```python
from build123d import *

# Parameters (mm, degrees)
SKETCH1_R          = 9.525
BODY_DEPTH         = 6
SKETCH2_R          = 1.5
SKETCH2_R_2        = 5.5
SKETCH2_R_3        = 1.75
HOLES_DEPTH        = 6
FILLET1_R          = 10
FILLET2_R          = 40
SKETCH3_R          = 3.175
CUT_EXTRUDE2_DEPTH = 3


with BuildPart() as part:
    # Sketch1 → Body (new body)
    with BuildSketch(Plane(origin=(0, 0, 0), x_dir=(1, 0, 0), z_dir=(0, 1, 0))):
        with BuildLine():
            Line((45, -55), (15.965110713, -96.240145236))
            ThreePointArc((15.965110713, -96.240145236), (0, -104.525), (-15.965110713, -96.240145236))
            Line((-15.965110713, -96.240145236), (-45, -55))
            Line((-45, -55), (-45, 55))
            Line((-45, 55), (45, 55))
            Line((45, 55), (45, -55))
        make_face()
        with Locations(Location((0, -85, 0), (0, 0, 270))):
            Circle(SKETCH1_R, mode=Mode.SUBTRACT)
    extrude(amount=BODY_DEPTH)

    # Sketch2 → Holes (cut)
    with BuildSketch(Plane(origin=(0, 6, 0), x_dir=(1, 0, 0), z_dir=(0, 1, 0))):
        with Locations(Location((6.273420837, 45, 0), (0, 0, 270))):
            Circle(SKETCH2_R)
        with Locations(Location((-8.726579163, 45, 0), (0, 0, 270))):
            Circle(SKETCH2_R)
        with Locations(Location((-1.226579163, 45, 0), (0, 0, 270))):
            Circle(SKETCH2_R_2)
        with Locations(Location((37.5, -57.5, 0), (0, 0, 270))):
            Circle(SKETCH2_R_3)
        with Locations(Location((-37.5, -57.5, 0), (0, 0, 270))):
            Circle(SKETCH2_R_3)
        with Locations(Location((-37.5, -12.5, 0), (0, 0, 270))):
            Circle(SKETCH2_R_3)
        with Locations(Location((37.5, -12.5, 0), (0, 0, 270))):
            Circle(SKETCH2_R_3)
    extrude(amount=-HOLES_DEPTH, mode=Mode.SUBTRACT)

    # Fillet1
    fillet1_edges = [part.edges().sort_by_distance(p)[0] for p in [
        (45, 3, 55),
        (-45, 3, 55),
    ]]
    fillet(fillet1_edges, radius=FILLET1_R)

    # Fillet2
    fillet2_edges = [part.edges().sort_by_distance(p)[0] for p in [
        (-45, 3, -55),
        (45, 3, -55),
    ]]
    fillet(fillet2_edges, radius=FILLET2_R)

    # Sketch3 → Cut-Extrude2 (cut)
    with BuildSketch(Plane(origin=(0, 6, 0), x_dir=(1, 0, 0), z_dir=(0, 1, 0))):
        with Locations(Location((-37.5, -12.5, 0), (0, 0, 270))):
            Circle(SKETCH3_R)
        with Locations(Location((37.5, -12.5, 0), (0, 0, 270))):
            Circle(SKETCH3_R)
        with Locations(Location((37.5, -57.5, 0), (0, 0, 270))):
            Circle(SKETCH3_R)
        with Locations(Location((-37.5, -57.5, 0), (0, 0, 270))):
            Circle(SKETCH3_R)
        with BuildLine():
            Line((-8.726579163, 50.5), (6.273420837, 50.5))
            ThreePointArc((6.273420837, 50.5), (11.773420837, 45), (6.273420837, 39.5))
            Line((6.273420837, 39.5), (-8.726579163, 39.5))
            ThreePointArc((-8.726579163, 39.5), (-14.226579163, 45), (-8.726579163, 50.5))
        make_face()
    extrude(amount=-CUT_EXTRUDE2_DEPTH, mode=Mode.SUBTRACT)


solid = part.part
```
Verification items for the finished model (mm, model axes). A direction names the side the tool comes from. Round coordinates to 2 decimals unless told otherwise and drop trailing zeros. Write each loop counter-clockwise with the first axis right and the second up, starting at its lowest first coordinate (ties: lowest second). Pieces come first, ordered by that corner, then holes.
1. Section check C-C on x = 1.5. Enter the section's corners in (y, z), plus the area to 3 significant figures.
2. Section check B-B on y = 1.05. State how many separate pieces and enclosed holes the cut face has, plus the area to 3 significant figures.
3. Draft check along Z on faces 3 (the flat face through (29.761, 2.958, 76.644)), 4 (the cylindrical face through (-14.225, 4.521, -44.879)), 5 (the cylindrical face through (-32.972, 3.042, -43.594)). Enter one of: +Z half, -Z half, draft (parallel to the pull), parting line (faces both ways), or undercut.
4. Access from +Z, -Z, +X, -X, +Y, -Y to the whole of each face (thin tool, end or side, straight path). Record for faces 1 (the flat face through (-1, 5, -50.5)), 2 (the cylindrical face through (35.79, 1.52, 12.12)).
5. Section check D-D on x = 24.5. Enter the section's corners in (y, z), plus the area to 3 significant figures.
6. Gauge pin test, flat ends, axial feed: P1, Ø1.5, axis at x = 26, y = 0.5, coming from the -Z side; P2, Ø4, axis at x = -37.5, z = 57.5, coming from the +Y side; P3, Ø1, axis at y = 1, z = 82, coming from the +X side. Record the tip position at first contact, or that the pin passes through.
7. Scan lines: L1, parallel to X at y = 1.6, z = 12.5; L2, parallel to X at y = 4.1, z = 12.5 (3 decimals); L3, parallel to Z at x = -2, y = 4.9. Record each from-to range of solid material in increasing order.
8. Section check A-A on z = 12.5. Enter the section's corners in (x, y) (3 decimals), plus the area to 3 significant figures.
Answer:
1. outline: (0, -55) - (6, -55) - (6, -50.5) - (3, -50.5) - (3, -49.78) - (0, -49.78) - close; (0, -40.22) - (3, -40.22) - (3, -39.5) - (6, -39.5) - (6, 75.59) - (0, 75.59) - close; (0, 94.41) - (6, 94.41) - (6, 104.47) - (0, 104.47) - close
1. area: 782 mm2
2. separate pieces: 1
2. enclosed holes: 8
2. area: 11,500 mm2
3. face 3: +Z half
3. face 4: undercut
3. face 5: -Z half
4. face 1: +Y
4. face 2: +Y, -Y
5. outline: (0, -49.92) - (6, -49.92) - (6, 84.12) - (0, 84.12) - close
5. area: 804 mm2
6. P1: stops at z = -49.5
6. P2: stops at y = 3
6. P3: stops at x = 26.34
7. L1: x = -45 to -39.25, -35.75 to 35.75, 39.25 to 45
7. L2: x = -45 to -40.675, -34.325 to 34.325, 40.675 to 45
7. L3: z = -55 to -50.5, -39.5 to 75.69, 94.31 to 104.42
8. outline: (-45, 0) - (-39.25, 0) - (-39.25, 3) - (-40.675, 3) - (-40.675, 6) - (-45, 6) - close; (-35.75, 0) - (35.75, 0) - (35.75, 3) - (34.325, 3) - (34.325, 6) - (-34.325, 6) - (-34.325, 3) - (-35.75, 3) - close; (39.25, 0) - (45, 0) - (45, 6) - (40.675, 6) - (40.675, 3) - (39.25, 3) - close
8. area: 481 mm2
